Check sheet for the modelled part. Datum: model origin and axes. Units: mm. A direction names the side the tool comes from. Round coordinates to 2 decimals unless told otherwise and drop trailing zeros. Loops run counter-clockwise (first coordinate to the right, second up) from the corner with the lowest first, then second, coordinate; pieces in that order, holes last. Notation, with made-up numbers: (-1.5, -26) -> (47.5, -26) arc R20 cw to (47.5, 3) -> close; hole circle Ø5 at (89.5, -11.75). An arc over 180 degrees is marked (long way). Use one line per item in the form item = value. Start each with the question number.
(1) Draft check along Y on faces 3 (the flat face through (76.5, -9, 5)), 4 (the flat face through (38, -18.1, 4)), 5 (the cylindrical face through (13.32, -7.935, 8.528)). Enter one of: released by +Y, released by -Y, zero draft, split by the parting line, or undercut.
(2) Material ranges on probe 1 along X at (y, z) = (-10.3, 1.4); probe 2 along X at (y, z) = (-10.3, 9.15); probe 3 along Y at (x, z) = (15.9, 3.55), recorded low to high. Write a range as [from, to].
(3) Sectioned sample at C-C (z = 4). Record the cut outline in (x, y).
(4) Set-up check for faces 1 (the cylindrical face through (11.85, -14.02, 2.47)), 2 (the cylindrical face through (63.94, -9.25, 8.53)): record each of +Z, -Z, +X, -X, +Y, -Y from which the full face is reachable in a straight line by a thin tool's end or side.
(5) Go/stop test with flat-tipped pins: pin 1 (2 mm diameter, centred on x = 60.5, y = -9.5, fed in from -Z); pin 2 (10 mm diameter, centred on x = 15.9, y = -10.3, fed in from -Z). Record where each tip stops, or that it passes through.
(6) Sectioned sample at A-A (y = -10.3). State how many separate pieces and enclosed holes the cut face has, and give its area (3 significant figures).
from build123d import *

# Parameters (mm, degrees)
F0_W     = 76.5
F0_H     = 18.1
F0_R     = 3.5
F1_DEPTH = 10.1
F2_R     = 5.5
F3_DEPTH = 7
F4_R     = 1.99999
F5_SIZE  = 2


# Not quite as in the source:
# - a fillet or chamfer is up to 0.001 mm smaller than in the source, because OpenCascade refuses the exact size
# - a feature names something its author has since deleted; it is built from what else it names


with BuildPart() as f1:
    # F0 (on Top) → F1 (new body)
    with BuildSketch(Plane.XY):
        with Locations((38.25, -9.05)):
            Rectangle(F0_W, F0_H)
        with Locations((15.9, -10.3)):
            Circle(F0_R, mode=Mode.SUBTRACT)
        with Locations((60.6, -10.3)):
            Circle(F0_R, mode=Mode.SUBTRACT)
    extrude(amount=F1_DEPTH)

    # F2 (on face) → F3 (cut)
    with BuildSketch(Plane(origin=(0, 0, 0), x_dir=(1, 0, 0), z_dir=(0, 0, -1))):
        with Locations((60.6, 10.3)):
            Circle(F2_R)
        with Locations((15.9, 10.3)):
            Circle(F2_R)
    extrude(amount=-F3_DEPTH, mode=Mode.SUBTRACT)

    # F4 (radius 2 in the source; OpenCascade refuses exactly that, so slightly less here)
    f4_edges = [f1.edges().sort_by_distance(p)[0] for p in [
        (55.1, -10.3, 7),
        (10.4, -10.3, 7),
    ]]
    fillet(f4_edges, radius=F4_R)

    # F5
    f5_edges = [f1.edges().sort_by_distance(p)[0] for p in [
        (38.25, -18.1, 10.1),
    ]]
    chamfer(f5_edges, length=F5_SIZE)


solid = f1.part
Checks:
q1.face_3 = zero draft
q1.face_4 = released by -Y
q1.face_5 = undercut
q2.probe_1 = [0, 10.4], [21.4, 55.1], [66.1, 76.5]
q2.probe_2 = [0, 12.4], [19.4, 57.1], [64.1, 76.5]
q2.probe_3 = [-18.1, -15.8], [-4.8, 0]
q3.outline = (0, -18.1) -> (76.5, -18.1) -> (76.5, 0) -> (0, 0) -> close; hole circle Ø11 at (15.9, -10.3); hole circle Ø11 at (60.6, -10.3)
q4.face_1 = -Z
q4.face_2 = +Z, -Z
q5.pin_1 = through
q5.pin_2 = 6.32
q6.separate_pieces = 3
q6.enclosed_holes = 0
q6.area = 579 mm2
